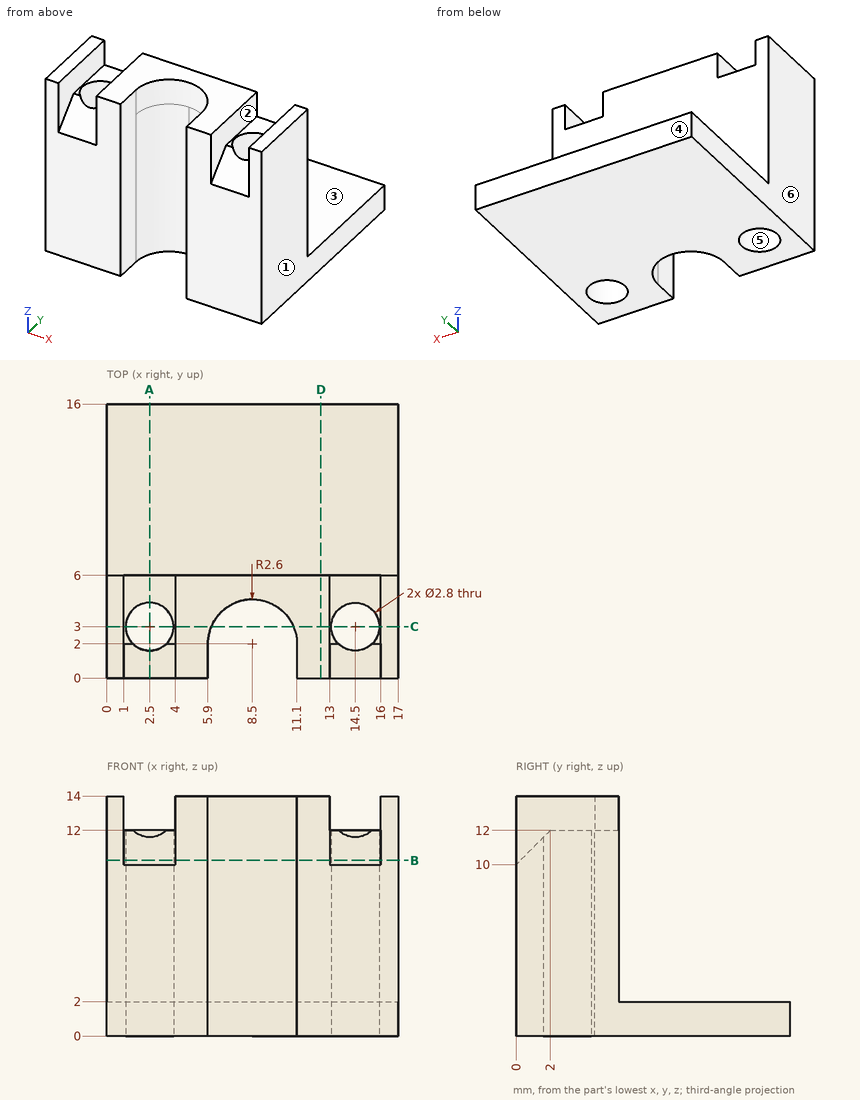
Geometry check sheet. Reference: drawing and pictorial views, mm from the part's lowest x, y, z. A direction names the side the tool comes from. Round coordinates to 2 decimals unless told otherwise and drop trailing zeros. Loops run counter-clockwise (first coordinate to the right, second up) from the corner with the lowest first, then second, coordinate; pieces in that order, holes last. Notation, with made-up numbers: (77, -13) - (119, -13) arc R11 ccw to (119, 3) - close; hole circle Ø1 at (86.5, -4). An arc over 180 degrees is marked (long way). Use a Markdown table: item, result. Add a question column.
1. Section check D-D, the plane x = 12.5. Record the boundary of the cut face in (y, z), plus the area to 3 significant figures.
2. Section check B-B, the plane z = 10.25. Record the boundary of the cut face in (x, y), plus the area to 3 significant figures.
3. Thickness scan on probe 1 along X at (y, z) = (1.5, 13.25); probe 2 along Y at (x, z) = (14.5, 5); probe 3 along X at (y, z) = (3, 4). Record the ranges inside material, lowest first. Write a range as [from, to].
4. Section check C-C, the plane y = 3. Record the boundary of the cut face in (x, z).
5. Release check for a two-part mould opening along X. For the marked faces 4, 5 and 6 record: released by +X, released by -X, zero draft, split by the parting line, or undercut.
6. Gauge pin test, flat ends, axial feed: pin 1 (4 mm diameter, centred on x = 12.5, y = 9.5, fed in from +Z); pin 2 (2.5 mm diameter, centred on x = 14.5, y = 4.5, fed in from +Z); pin 3 (3 mm diameter, centred on x = 14.5, z = 4, fed in from +Y). Record the tip position at first contact, or that the pin passes through.
7. Section check A-A, the plane x = 2.5. Record the boundary of the cut face in (y, z), plus the area to 3 significant figures.
8. Access from +Z, -Z, +X, -X, +Y, -Y to the whole of each face (thin tool, end or side, straight path). Record for the marked faces 1, 2 and 3.
Checks:
| question | item | result |
|---|---|---|
| 1 | outline | (0, 0) - (16, 0) - (16, 2) - (6, 2) - (6, 14) - (0, 14) - close |
| 1 | area | 104 mm^2 |
| 2 | outline | (0, 0) - (1, 0) - (1, 0.25) - (4, 0.25) - (4, 0) - (5.9, 0) - (5.9, 2) arc R2.6 cw to (11.1, 2) - (11.1, 0) - (13, 0) - (13, 0.25) - (16, 0.25) - (16, 0) - (17, 0) - (17, 6) - (0, 6) - close; hole circle Ø2.8 at (2.5, 3); hole circle Ø2.8 at (14.5, 3) |
| 2 | area | 67.2 mm^2 |
| 3 | probe 1 | x = [0, 1], [4, 5.9], [11.1, 13], [16, 17] |
| 3 | probe 2 | y = [0, 1.6], [4.4, 6] |
| 3 | probe 3 | x = [0, 1.1], [3.9, 6.1], [10.9, 13.1], [15.9, 17] |
| 4 | outline | (0, 0) - (1.1, 0) - (1.1, 12) - (1, 12) - (1, 14) - (0, 14) - close; (3.9, 0) - (6.1, 0) - (6.1, 14) - (4, 14) - (4, 12) - (3.9, 12) - close; (10.9, 0) - (13.1, 0) - (13.1, 12) - (13, 12) - (13, 14) - (10.9, 14) - close; (15.9, 0) - (17, 0) - (17, 14) - (16, 14) - (16, 12) - (15.9, 12) - close |
| 5 | face 4 | zero draft |
| 5 | face 5 | undercut |
| 5 | face 6 | released by -X |
| 6 | pin 1 | stops at z = 2 |
| 6 | pin 2 | stops at z = 12 |
| 6 | pin 3 | stops at y = 6 |
| 7 | outline | (0, 0) - (1.6, 0) - (1.6, 11.6) - (0, 10) - close; (4.4, 0) - (16, 0) - (16, 2) - (6, 2) - (6, 12) - (4.4, 12) - close |
| 7 | area | 56.5 mm^2 |
| 8 | face 1 | +Z, -Z, +X, +Y, -Y |
| 8 | face 2 | +Z, -Y |
| 8 | face 3 | +Z, +X, -X, +Y |
